from build123d import *

# Parameters (mm, degrees)
F2_R = 5.08
F3_R = 5.08
F4_T = -2.54


with BuildPart() as f1:
    # F0 (on Front) → F1 (revolve)
    with BuildSketch(Plane.XZ):
        Polygon((0, 32.165237), (-9.322633, 32.165237), (-9.322633, 24.169475), (0, 24.169475), (9.322633, 24.169475), (9.322633, 32.165237), align=None)
    revolve(axis=Axis((0.987695, 0, 0), (1, 0, 0)))

    # F2
    f2_edges = [f1.edges().sort_by_distance(p)[0] for p in [
        (9.322633, 0, -32.165237),
    ]]
    fillet(f2_edges, radius=F2_R)

    # F3
    f3_edges = [f1.edges().sort_by_distance(p)[0] for p in [
        (-9.322633, 0, -32.165237),
    ]]
    fillet(f3_edges, radius=F3_R)

    # F4
    f4_openings = [f1.faces().sort_by_distance(p)[0] for p in [
        (0, 0, -24.169475),
    ]]
    offset(amount=F4_T, openings=f4_openings)


solid = f1.part
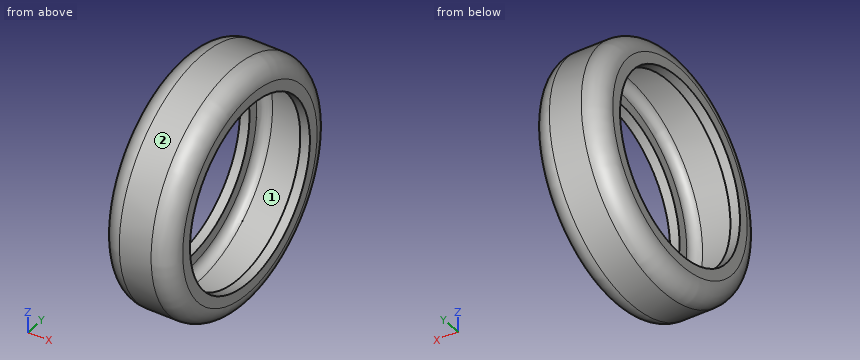
Verification items for the finished model (mm, model axes). Face numbers are marked on the shaded views. Coordinates: 2 decimals unless noted, no trailing zeros. Loops run counter-clockwise (first coordinate to the right, second up) from the corner with the lowest first, then second, coordinate; pieces in that order, holes last. Notation, with made-up numbers: (32, 17) -> (86, 17) arc R26 cw to (86, 33) -> close; hole circle Ø7 at (10.25, 18.5). An arc over 180 degrees is marked (long way). Write each question's results on one line, items separated by ' | '.
Item 1: Section check C-C, the plane x = -3.25. Enter the section's corners in (y, z).
Found:
outline: circle Ø64.33 at (0, 0); hole circle Ø59.25 at (0, 0)
Item 2: Section check A-A, the plane z = 0. Enter the section's corners in (x, y), plus the area to 3 significant figures.
Found:
outline: (-9.32, -27.09) arc R5.08 ccw to (-4.24, -32.17) -> (4.24, -32.17) arc R5.08 ccw to (9.32, -27.09) -> (9.32, -24.17) -> (6.78, -24.17) -> (6.78, -27.09) arc R2.54 cw to (4.24, -29.63) -> (-4.24, -29.63) arc R2.54 cw to (-6.78, -27.09) -> (-6.78, -24.17) -> (-9.32, -24.17) -> close; (-9.32, 24.17) -> (-6.78, 24.17) -> (-6.78, 27.09) arc R2.54 cw to (-4.24, 29.63) -> (4.24, 29.63) arc R2.54 cw to (6.78, 27.09) -> (6.78, 24.17) -> (9.32, 24.17) -> (9.32, 27.09) arc R5.08 ccw to (4.24, 32.17) -> (-4.24, 32.17) arc R5.08 ccw to (-9.32, 27.09) -> close | area: 134 mm2
Item 3: Material ranges on L1, parallel to X at y = -24.5, z = -4.5; L2, parallel to Z at x = -1, y = 0; L3, parallel to Z at x = -1.25, y = -16, recorded low to high.
Found:
L1: x = -9.32 to -6.78, 6.78 to 9.32 | L2: z = -32.17 to -29.63, 29.63 to 32.17 | L3: z = -27.9 to -24.93, 24.93 to 27.9
Item 4: Gauge pin test, flat ends, axial feed: pin 1 (2 mm diameter, centred on x = 4, y = -7.5, fed in from -Z); pin 2 (10 mm diameter, centred on x = 5.5, y = 6, fed in from -Z); pin 3 (2 mm diameter, centred on x = -5.5, y = 25, fed in from +Z); pin 4 (1.5 mm diameter, centred on y = -8.5, z = 21.5, fed in from -X). Record the tip position at first contact, or that the pin passes through.
Found:
pin 1: stops at z = -31.5 | pin 2: stops at z = -32.14 | pin 3: stops at z = 21.23 | pin 4: passes through
Item 5: Mould release check, pull along Y, two halves, no side actions. Record for the marked faces 1 and 2: +Y half, -Y half, draft (parallel to the pull), parting line (faces both ways), or undercut.
Found:
face 1: undercut | face 2: parting line
